from build123d import *

# Parameters (mm, degrees)
F0_R     = 2.5
F1_DEPTH = 5


with BuildPart() as f1:
    # F0 (on Front) → F1 (new body)
    with BuildSketch(Plane.XZ):
        with BuildLine():
            Line((0, 4), (-25, 4))
            ThreePointArc((-25, 4), (-29, 0), (-25, -4))
            Line((-25, -4), (0, -4))
            Line((0, -4), (0, 4))
        make_face()
        with Locations((-25, 0)):
            Circle(F0_R, mode=Mode.SUBTRACT)
        with BuildLine():
            Line((25, 4), (0, 4))
            Line((0, 4), (0, -4))
            Line((0, -4), (25, -4))
            ThreePointArc((25, -4), (29, 0), (25, 4))
        make_face()
        with Locations((25, 0)):
            Circle(F0_R, mode=Mode.SUBTRACT)
    extrude(amount=F1_DEPTH)


solid = f1.part
Input: part model. Units: mm. Frame: model coordinates. Coordinates: 2 decimals unless noted, no trailing zeros. Order: outer loops, then holes, each group sorted by start corner. A loop starts at its lowest first (then second) coordinate and runs counter-clockwise, first axis right, second up. Notation, with made-up numbers: M 36,-5 L 70,-5 A22 cw 70,11 Z; hole C 40.5,77.25 d5. An arc over 180 degrees is marked long. Write item = value, one per line. Start each with the question number.
(1) Line query: line 1 along Z through (x, y) = (25, -3.75); line 2 along X through (y, z) = (-3.4, 0.75); line 3 along X through (y, z) = (-2.4, -0.25). Output: solid intervals per line, ascending. Write a range as [from, to].
(2) Pull-direction query (Z, two-part tool) for faces 1 (the cylindrical face through (-29, -2, 0)), 2 (the cylindrical face through (-27.5, -2.5, 0.1)), 3 (the flat face through (0, 0, 0)), 4 (the cylindrical face through (22.5, -2.5, 0.1)); classes: released by +Z, released by -Z, zero draft, split by the parting line, or undercut.
(3) First-contact query: P1, Ø1.5, axis at y = -2.5, z = 3, coming from the -X side; P2, Ø2, axis at y = -4, z = 2, coming from the +X side; P3, Ø3, axis at x = 25, z = 0, coming from the -Y side. Flat tips, straight axial feed; report the tip coordinate or a pass-through.
(4) Section B-B on y = -0.65. Output: boundary loops of the cut face in (x, z).
(5) Section A-A on z = 0. Output: boundary loops of the cut face in (x, y).
Result set:
q1.line_1 = [-4, -2.5], [2.5, 4]
q1.line_2 = [-28.93, -27.38], [-22.62, 22.62], [27.38, 28.93]
q1.line_3 = [-28.99, -27.49], [-22.51, 22.51], [27.49, 28.99]
q2.face_1 = split by the parting line
q2.face_2 = undercut
q2.face_3 = zero draft
q2.face_4 = undercut
q3.P1 = -28.31
q3.P2 = 28.87
q3.P3 = through
q4.outline = M -25,-4 L 25,-4 A4 ccw 25,4 L -25,4 A4 ccw Z; hole C -25,0 d5; hole C 25,0 d5
q5.outline = M -29,-5 L -27.5,-5 L -27.5,0 L -29,0 Z; M -22.5,-5 L 22.5,-5 L 22.5,0 L -22.5,0 Z; M 27.5,-5 L 29,-5 L 29,0 L 27.5,0 Z
